Check sheet for the modelled part. Datum: model origin and axes. Units: mm. A direction names the side the tool comes from. Round coordinates to 2 decimals unless told otherwise and drop trailing zeros. Order: outer loops, then holes, each group sorted by start corner. A loop starts at its lowest first (then second) coordinate and runs counter-clockwise, first axis right, second up.
Autodesk Inventor part; units mm, degrees
ref_plane "YZ Plane" through (0, 0, 0) normal (1, 0, 0) x (0, 1, 0)
ref_plane "XZ Plane" through (0, 0, 0) normal (0, 1, 0) x (-1, 0, 0)
ref_plane "XY Plane" through (0, 0, 0) normal (0, 0, 1) x (1, 0, 0)
sketch "Sketch2" plane through (0, 0, 0) normal (0, 0, 1) x (1, 0, 0)
  line L0 (0, 0) -> (6.604, 0)
  line L1 (6.604, 0) -> (6.604, 12.7)
  line L2 (6.604, 12.7) -> (0, 12.7)
  line L3 (0, 12.7) -> (0, 0)
  dimension "d0" = 6.604
  dimension "d1" = 12.7
extrude "Extrusion1" add sketch "Sketch2" along normal blind 9.398
sketch "Sketch3" plane through (0, 0, 9.398) normal (0, 0, 1) x (1, 0, 0)
  line L0 (6.604, 12.7) -> (0, 12.7)
  line L1 (3.302, 9.398) -> (3.302, 3.556) construction
  circle A0 centre (3.302, 6.477) radius 2.921
  point P0 (0, 0)
  dimension "d5" = 5.842
extrude "Extrusion2" add sketch "Sketch3" along normal blind 8.509
sketch "Sketch4" plane through (3.302, 6.477, 17.907) normal (0, 0, 1) x (1, 0, 0)
  circle A0 centre (0, 0) radius 1.27
  point P0 (-3.302, -6.477)
  dimension "d8" = 2.54
extrude "Extrusion3" add sketch "Sketch4" along normal blind 10.414
properties part number "msheehan_switch"
Item 1: Go/stop test with flat-tipped pins: P1, Ø1, axis at y = 7.5, z = 20, coming from the +X side; P2, Ø6, axis at y = 7.5, z = 25, coming from the +X side; P3, Ø1.5, axis at x = 0.5, y = 4.5, coming from the +Z side. Record where each tip stops, or that it passes through.
Answer:
P1: stops at x = 4.46
P2: stops at x = 4.57
P3: stops at z = 17.91
Item 2: Access from +Z, -Z, +X, -X, +Y, -Y to the whole of each face (thin tool, end or side, straight path). Record for faces 1 (the flat face through (6.604, 6, 5)), 2 (the flat face through (1.8, 3.6, 9.398)).
Answer:
face 1: +Z, -Z, +X, +Y, -Y
face 2: +Z
Item 3: Sectioned sample at B-B (y = 5.5). Record the cut outline in (x, z).
Answer:
outline: (0, 0) - (6.6, 0) - (6.6, 9.4) - (6.05, 9.4) - (6.05, 17.91) - (4.11, 17.91) - (4.11, 28.32) - (2.49, 28.32) - (2.49, 17.91) - (0.55, 17.91) - (0.55, 9.4) - (0, 9.4) - close
Item 4: Scan lines: line 1 along Z through (x, y) = (3, 3); line 2 along Z through (x, y) = (2, 6.5); line 3 along Y through (x, z) = (3.5, 15.5). Record each from-to range of solid material in increasing order.
Answer:
line 1: z = 0 to 9.4
line 2: z = 0 to 17.91
line 3: y = 3.56 to 9.39
Item 5: Sectioned sample at C-C (z = 20). Record the cut outline in (x, y).
Answer:
outline: circle Ø2.54 at (3.3, 6.48)
Item 6: Sectioned sample at D-D (y = 11.75). Record the cut outline in (x, z).
Answer:
outline: (0, 0) - (6.6, 0) - (6.6, 9.4) - (0, 9.4) - close
Item 7: Sectioned sample at A-A (x = 3.25). Record the cut outline in (y, z), and give its area (3 significant figures).
Answer:
outline: (0, 0) - (12.7, 0) - (12.7, 9.4) - (9.4, 9.4) - (9.4, 17.91) - (7.75, 17.91) - (7.75, 28.32) - (5.21, 28.32) - (5.21, 17.91) - (3.56, 17.91) - (3.56, 9.4) - (0, 9.4) - close
area: 195 mm2
